The model under review builds one solid part; all positions refer to its coordinate system, in mm. Round coordinates to 2 decimals unless told otherwise and drop trailing zeros. Write each loop counter-clockwise with the first axis right and the second up, starting at its lowest first coordinate (ties: lowest second). Pieces come first, ordered by that corner, then holes. Notation, with made-up numbers: (-20, 41) - (5, 41) arc R18 ccw to (5, 66) - close; hole circle Ø2 at (89.5, -22.5). An arc over 180 degrees is marked (long way). Return JSON: item names as keys, results as strings.
Autodesk Inventor part; units mm, degrees
ref_plane "YZ Plane" through (0, 0, 0) normal (1, 0, 0) x (0, 1, 0)
ref_plane "XZ Plane" through (0, 0, 0) normal (0, 1, 0) x (-1, 0, 0)
ref_plane "XY Plane" through (0, 0, 0) normal (0, 0, 1) x (1, 0, 0)
sketch "Sketch1" plane through (0, 0, 0) normal (0, 0, 1) x (1, 0, 0)
  point P0 (0, 0)
sketch "Sketch2" plane through (0, 0, 0) normal (0, 0, 1) x (1, 0, 0)
  line L0 (0, 0) -> (127, 0)
  line L1 (127, 0) -> (127, 304.8)
  line L2 (127, 304.8) -> (0, 304.8)
  line L3 (0, 304.8) -> (0, 0)
  circle A0 centre (17.338, 279.4) radius 3.9687
  circle A1 centre (109.662, 279.4) radius 3.9687
  circle A2 centre (17.338, 25.4) radius 3.9688
  circle A3 centre (109.662, 25.4) radius 3.9688
  dimension "d0" = 127
  dimension "d1" = 304.8
  dimension "d2" = 7.9375
  dimension "d3" = 25.4
  dimension "d4" = 17.338
  dimension "d5" = 7.9375
  dimension "d6" = 17.338
  dimension "d7" = 25.4
  dimension "d8" = 7.9375
  dimension "d9" = 17.338
  dimension "d10" = 25.4
  dimension "d11" = 7.9375
  dimension "d12" = 17.338
  dimension "d13" = 25.4
extrude "Extrusion1" add sketch "Sketch2" along normal blind 12.7
sketch "Sketch3" plane through (0, 0, 12.7) normal (0, 0, 1) x (1, 0, 0)
  line L0 (127, 304.8) -> (0, 304.8)
  line L1 (0, 0) -> (127, 0)
  line L2 (0, 304.8) -> (0, 0)
  line L3 (127, 0) -> (127, 304.8)
  circle A0 centre (46, 232.918) radius 0.635
  circle A1 centre (63.5, 250.4307) radius 0.635
  circle A2 centre (63.5, 215.4307) radius 0.635
  circle A3 centre (81, 232.918) radius 0.635
  circle A4 centre (63.5, 169.4307) radius 14.2875
  circle A5 centre (63.5, 169.4307) radius 23.8252
  point P0 (63.5, 232.9307)
  point P1 (68.244, 192.7788)
  point P2 (45.652, 185.2132)
  point P3 (40.9079, 161.8651)
  point P4 (58.756, 146.0826)
  point P5 (81.348, 153.6482)
  point P6 (86.0921, 176.9963)
  dimension "d18" = 63.5
  dimension "d19" = 63.5
  dimension "d31" = 1.27
  dimension "d32" = 1.27
  dimension "d33" = 1.27
  dimension "d34" = 1.27
  dimension "d45" = 34.9999
  dimension "d46" = 17.5
  dimension "d47" = 17.5
  dimension "d48" = 17.5
  dimension "d49" = 28.575
  dimension "d50" = 169.4307
  dimension "d53" = 23.8252
  dimension "d56" = 360
  dimension "d66" = 63.5
  dimension "d67" = 63.5
  dimension "d68" = 63.5
  dimension "d69" = 63.5
  dimension "d70" = 71.8693
  dimension "d71" = 71.882
  dimension "d72" = 71.882
hole "Hole1" at (63.5, 232.9307, 12.7) direction (0, 0, -1) diameter 1.27 end through all
extrude "Extrusion2" cut sketch "Sketch3" against normal blind 25.4 contours A0 | A1 | A2 | A3
extrude "Extrusion3" cut sketch "Sketch3" against normal blind 25.4 contours A4
hole "Hole2" at (68.244, 192.7788, 12.7) at (45.652, 185.2132, 12.7) at (40.9079, 161.8651, 12.7) at (58.756, 146.0826, 12.7) at (81.348, 153.6482, 12.7) at (86.0921, 176.9963, 12.7) direction (0, 0, -1) diameter 5.08 end through all
(1) Mouldability with a two-part tool opening along X and no side actions: class faces 1 (the flat face through (63, 155, 0)), 2 (the cylindrical face through (113.33, 26.92, 6.26)), 3 (the cylindrical face through (43.94, 187.09, 6.26)), 4 (the flat face through (0, 155, 6)) as released by +X, released by -X, zero draft, split by the parting line, or undercut.
Filled in:
{"face 1": "zero draft", "face 2": "undercut", "face 3": "undercut", "face 4": "released by -X"}
(2) Wall thickness on line 1 (Y direction, x = 63.5, z = 9.25); line 2 (Y direction, x = 63, z = 9.5); line 3 (Y direction, x = 57, z = 10.75): over which ranges is each line inside the solid? List them lowest first.
Filled in:
{"line 1": "y = 0 to 155.14, 183.72 to 214.8, 216.07 to 232.3, 233.57 to 249.8, 251.07 to 304.8", "line 2": "y = 0 to 155.15, 183.71 to 215.04, 215.82 to 232.54, 233.32 to 250.04, 250.82 to 304.8", "line 3": "y = 0 to 144.25, 147.92 to 156.71, 182.15 to 304.8"}
(3) Add section B-B (z = 10.25). Give the number of separate pieces and of enclosed holes in the cut face, plus the area to 3 significant figures.
Filled in:
{"separate pieces": "1", "enclosed holes": "16", "area": "37,700 mm2"}
(4) Add section A-A (y = 279.4). Write out the cut boundary in (x, z), plus the area to 3 significant figures.
Filled in:
{"outline": "(0, 0) - (13.37, 0) - (13.37, 12.7) - (0, 12.7) - close; (21.31, 0) - (105.69, 0) - (105.69, 12.7) - (21.31, 12.7) - close; (113.63, 0) - (127, 0) - (127, 12.7) - (113.63, 12.7) - close", "area": "1,410 mm2"}
